from build123d import *

# Parameters (mm, degrees)
BOSS_EXTRUDE1_DEPTH                    = 22
CBORE_FOR_M5_HEX_HEAD_BOLT1_AT_2_COUNT = 2
CBORE_FOR_M5_HEX_HEAD_BOLT1_AT_2_PITCH = 28
BOSS_EXTRUDE2_DEPTH                    = 3
CUT_EXTRUDE1_DEPTH                     = 87.362098425
FILLET2_R                              = 10
FILLET3_R                              = 10


with BuildPart() as part:
    # Sketch1 → Boss-Extrude1 (new, symmetric)
    with BuildSketch(Plane.XY):
        Polygon((-41.920628378, 5.592699718), (38.079371622, 5.592699718), (38.079371622, -6.407300282), (-48.848831609, -6.407300282), (-74.312933224, 37.697817484), (-63.920628378, 43.697817484), align=None)
    extrude(amount=BOSS_EXTRUDE1_DEPTH, both=True)

    # Sketch3 → CBORE for M5 Hex Head Bolt1 (revolve, cut)
    with BuildSketch(Plane(origin=(-58.920628378, 35.037563446, -14), x_dir=(-0.4999999999999982, 0.8660254037844396, 0), z_dir=(0, 0, 1))):
        Polygon((0, 0), (0, 34.052558883), (2.75, 34.052558883), (2.75, 3.58), (6.12, 3.58), (6.12, 0.024), (6.144, 0), align=None)
    cbore_for_m5_hex_head_bolt1 = revolve(axis=Axis((-53.421367064, 38.212563446, -14), (-0.8660254037844397, -0.4999999999999983, 0)), mode=Mode.SUBTRACT)

    # CBORE for M5 Hex Head Bolt1 at 2: CBORE for M5 Hex Head Bolt1 ×2
    with Locations(*[(0, 0, i * CBORE_FOR_M5_HEX_HEAD_BOLT1_AT_2_PITCH) for i in range(1, CBORE_FOR_M5_HEX_HEAD_BOLT1_AT_2_COUNT)]):
        add(cbore_for_m5_hex_head_bolt1, mode=Mode.SUBTRACT)

    # Sketch4 → Boss-Extrude2 (add, symmetric)
    with BuildSketch(Plane.XY):
        Polygon((-63.920628378, 43.697817484), (-41.920628378, 5.592699718), (-16.920628378, 5.592699718), align=None)
    extrude(amount=BOSS_EXTRUDE2_DEPTH, both=True)

    # Sketch5 → Cut-Extrude1 (cut, through all)
    with BuildSketch(Plane(origin=(0, 5.592699718, 0), x_dir=(1, 0, 0), z_dir=(0, 1, 0))):
        with BuildLine():
            ThreePointArc((16.079371622, 22), (31.635720831, 15.556349163), (38.079371622, -6.4e-08))
            Line((38.079371622, -6.4e-08), (38.079371622, 22))
            Line((38.079371622, 22), (16.079371622, 22))
        make_face()
        with BuildLine():
            ThreePointArc((38.079371622, -6.4e-08), (31.635720785, -15.556349209), (16.079371622, -22))
            Line((16.079371622, -22), (38.079371622, -22))
            Line((38.079371622, -22), (38.079371622, -6.4e-08))
        make_face()
        with BuildLine():
            Line((-8.920628378, -6), (16.079371622, -6))
            ThreePointArc((16.079371622, -6), (22.079371622, 0), (16.079371622, 6))
            Line((16.079371622, 6), (-8.920628378, 6))
            ThreePointArc((-8.920628378, 6), (-14.920628378, 0), (-8.920628378, -6))
        make_face()
    extrude(amount=-CUT_EXTRUDE1_DEPTH, mode=Mode.SUBTRACT)

    # Fillet2
    fillet2_edges = [part.edges().sort_by_distance(p)[0] for p in [
        (-69.116780801, 40.697817484, 22),
    ]]
    fillet(fillet2_edges, radius=FILLET2_R)

    # Fillet3
    fillet3_edges = [part.edges().sort_by_distance(p)[0] for p in [
        (-69.116780801, 40.697817484, -22),
    ]]
    fillet(fillet3_edges, radius=FILLET3_R)


solid = part.part
Can you work these out from the model? Positions are in its coordinate system, mm. A direction names the side the tool comes from. Coordinates: 2 decimals unless noted, no trailing zeros. Order: outer loops, then holes, each group sorted by start corner. A loop starts at its lowest first (then second) coordinate and runs counter-clockwise, first axis right, second up. Notation, with made-up numbers: (58, -11) -> (102, -11) arc R10 ccw to (102, -4) -> close; hole circle Ø8 at (46, -22). An arc over 180 degrees is marked (long way). Use one line per item in the form item = value.
Q1. Imagine slicing it at C-C, the plane y = 25. List the corners of the cut face in (x, z) for me, then the cut area to 3 significant figures.
From the geometry:
outline = (-66.98, -22) -> (-53.13, -22) -> (-53.13, -3) -> (-40.86, -3) -> (-40.86, 3) -> (-53.13, 3) -> (-53.13, 22) -> (-66.98, 22) -> close
area = 683 mm²
Q2. Imagine slicing it at B-B, the plane x = -36. List the corners of the cut face in (y, z) for me.
From the geometry:
outline = (-6.41, -22) -> (5.59, -22) -> (5.59, -3) -> (21.06, -3) -> (21.06, 3) -> (5.59, 3) -> (5.59, 22) -> (-6.41, 22) -> close
Q3. Will these pins go through, and if not, where does the flat tip stop? P1, Ø2, axis at x = -37.5, z = 2.5, coming from the +Y side; P2, Ø5, axis at x = -35.5, z = -9.5, coming from the +Y side; P3, Ø5, axis at y = 29, z = 17.5, coming from the +X side.
From the geometry:
P1 = 23.09
P2 = 5.59
P3 = -53.99
Q4. Which directions (+Z, -Z, +X, -X, +Y, -Y) give clear straight access to the entire face, cutting with the end or side of a thin tool? Please do faces 1 (the face through (-2, 5.593, -9)), 2 (the face through (22.078, -0.323, 0.132)), 3 (the face through (-41, 18, -3)), 4 (the face through (-61.38, 32.14, 16.63)).
From the geometry:
face_1 = +X, +Y
face_2 = +Y, -Y
face_3 = -Z, +X, +Y
face_4 = none
Q5. Imagine slicing it at A-A, the plane y = 2. List the corners of the cut face in (x, z) for me.
From the geometry:
outline = (-53.7, -22) -> (16.08, -22) arc R22 ccw to (16.08, 22) -> (-53.7, 22) -> close; hole (-8.92, -6) -> (16.08, -6) arc R6 ccw to (16.08, 6) -> (-8.92, 6) arc R6 ccw to start
Q6. We'd pull the mould along Z, two halves only. Please class faces 5 (the face through (4, 0, -6)), 6 (the face through (-69.19, 40.656, 0.168)), 7 (the face through (-67.54, 38.136, 19.148)): released by +Z, released by -Z, zero draft, split by the parting line, or undercut.
From the geometry:
face_5 = undercut
face_6 = zero draft
face_7 = released by +Z
Q7. I need wall thicknesses on L1, parallel to Z at x = 14, y = -2.5; L2, parallel to Z at x = -38.5, y = 19; L3, parallel to Y at x = -17.5, z = -4. Which ranges of each line are inside material? Lowest first, please.
From the geometry:
L1 = -22 to -6, 6 to 22
L2 = -3 to 3
L3 = -6.41 to 5.59
